```python
from build123d import *

# Parameters (mm, degrees)
F0_R     = 25
F1_DEPTH = 200
F2_R     = 20
F3_DEPTH = 40
F4_R     = 14
F5_DEPTH = 26.95
F7_DEPTH = 25
F8_SIZE  = 2


with BuildPart() as f1:
    # F0 (on Top) → F1 (new body, symmetric)
    with BuildSketch(Plane.XY):
        Circle(F0_R)
    extrude(amount=F1_DEPTH, both=True)

    # F2 (on face) → F3 (join)
    with BuildSketch(Plane.XY.offset(200)):
        Circle(F2_R)
    extrude(amount=F3_DEPTH)

    # F4 (on face) → F5 (join)
    with BuildSketch(Plane(origin=(0, 0, -200), x_dir=(1, 0, 0), z_dir=(0, 0, -1))):
        Circle(F4_R)
    extrude(amount=F5_DEPTH)

    # F6 (on Front) → F7 (cut, symmetric)
    with BuildSketch(Plane.XZ):
        with BuildLine():
            ThreePointArc((6.5, -209.5), (0, -203), (-6.5, -209.5))
            Line((-6.5, -209.5), (-6.5, -211.5))
            ThreePointArc((-6.5, -211.5), (0, -218), (6.5, -211.5))
            Line((6.5, -211.5), (6.5, -209.5))
        make_face()
    extrude(amount=F7_DEPTH, both=True, mode=Mode.SUBTRACT)

    # F8
    f8_edges = [f1.edges().sort_by_distance(p)[0] for p in [
        (-14, 0, -226.95),
    ]]
    chamfer(f8_edges, length=F8_SIZE)


solid = f1.part
```
Model file for the job. Use its own axes, mm. A direction names the side the tool comes from. Give positions to 0.01 mm unless a question says otherwise; leave off trailing zeros. Write each loop counter-clockwise with the first axis right and the second up, starting at its lowest first coordinate (ties: lowest second). Pieces come first, ordered by that corner, then holes. Notation, with made-up numbers: (71, -37) -> (98, -37) arc R16 cw to (98, -22) -> close; hole circle Ø11 at (-3, -31). An arc over 180 degrees is marked (long way). Use CSV: the item, a comma, the result in double quotes. Start each with the question number.
1) Two-plate mould, pull along Z, no slides. Class faces 1 (the cylindrical face through (0, 0, -218)), 2 (the flat face through (0, 0, 240)), 3 (the cylindrical face through (-4.336, -19.524, 219.72)), 4 (the cylindrical face through (0, 0, -203)): released by +Z, released by -Z, zero draft, split by the parting line, or undercut.
2) Cut at C-C on z = -150.5. List the corners of the cut face in (x, y).
3) Tool access for faces 5 (the flat face through (0, 0, -226.95)), 6 (the flat face through (-11, 17, 200)), 7 (the cylindrical face through (13.35, -4.21, -212.3)): list every direction of +Z, -Z, +X, -X, +Y, -Y with a clear straight run to the whole face (end or side of a thin tool).
4) Drill centre lines: L1, parallel to Z at x = 0.5, y = 2; L2, parallel to Z at x = 1, y = -17; L3, parallel to Z at x = 2.5, y = 13.5. Where is each one in solid material? Low to high.
5) Pin check, flat tips, straight feed: P1, Ø6, axis at x = -13, y = 18.5, coming from the -Z side; P2, Ø1.5, axis at x = 7.5, z = -115.5, coming from the -Y side; P3, Ø1.5, axis at y = -17.5, z = 87.5, coming from the -X side. Stop position of each tip, or through.
6) Cut at B-B on y = 0. List the corners of the cut face in (x, z).
7) Cut at A-A on x = 0. List the corners of the cut face in (y, z), plus the area to 3 significant figures.
Final values:
1,face 1,"undercut"
1,face 2,"released by +Z"
1,face 3,"zero draft"
1,face 4,"undercut"
2,outline,"circle Ø50 at (0, 0)"
3,face 5,"-Z, +X, -X, +Y, -Y"
3,face 6,"+Z"
3,face 7,"-Z"
4,L1,"z = -226.95 to -217.98, -203.02 to 240"
4,L2,"z = -200 to 240"
4,L3,"z = -225.22 to -217.5, -203.5 to 240"
5,P1,"stops at z = -200"
5,P2,"stops at y = -24.07"
5,P3,"stops at x = -18.56"
6,outline,"(-25, -200) -> (-14, -200) -> (-14, -224.95) -> (-12, -226.95) -> (12, -226.95) -> (14, -224.95) -> (14, -200) -> (25, -200) -> (25, 200) -> (20, 200) -> (20, 240) -> (-20, 240) -> (-20, 200) -> (-25, 200) -> close; hole (-6.5, -211.5) arc R6.5 ccw to (6.5, -211.5) -> (6.5, -209.5) arc R6.5 ccw to (-6.5, -209.5) -> close"
7,outline,"(-25, -200) -> (-14, -200) -> (-14, -203) -> (14, -203) -> (14, -200) -> (25, -200) -> (25, 200) -> (20, 200) -> (20, 240) -> (-20, 240) -> (-20, 200) -> (-25, 200) -> close; (-14, -224.95) -> (-12, -226.95) -> (12, -226.95) -> (14, -224.95) -> (14, -218) -> (-14, -218) -> close"
7,area,"21,900 mm2"
